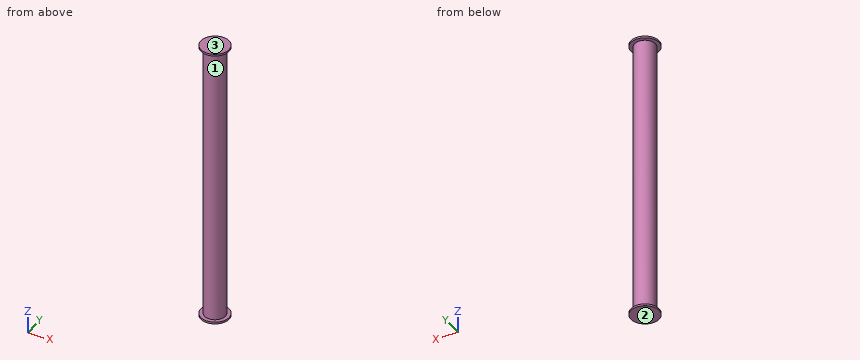
from build123d import *

# Parameters (mm, degrees)
SKETCH1_R           = 5.5
BOSS_EXTRUDE1_DEPTH = 150
SKETCH2_R           = 7.5
BOSS_EXTRUDE2_DEPTH = 1
SKETCH3_R           = 7.5
BOSS_EXTRUDE3_DEPTH = 1


with BuildPart() as part:
    # Sketch1 → Boss-Extrude1 (new body)
    with BuildSketch(Plane.XY):
        Circle(SKETCH1_R)
    extrude(amount=BOSS_EXTRUDE1_DEPTH)

    # Sketch2 → Boss-Extrude2 (add)
    with BuildSketch(Plane(origin=(0, 0, 0), x_dir=(-1, 0, 0), z_dir=(0, 0, -1))):
        Circle(SKETCH2_R)
    extrude(amount=BOSS_EXTRUDE2_DEPTH)

    # Sketch3 → Boss-Extrude3 (add)
    with BuildSketch(Plane.XY.offset(150)):
        Circle(SKETCH3_R)
    extrude(amount=BOSS_EXTRUDE3_DEPTH)


solid = part.part
Could you check a few things on this model? Use its own coordinates, in mm. Face numbers are marked on the shaded views. Give positions to 0.01 mm unless a question says otherwise; leave off trailing zeros. Order: outer loops, then holes, each group sorted by start corner. A loop starts at its lowest first (then second) coordinate and runs counter-clockwise, first axis right, second up. Notation, with made-up numbers: (38.25, -6.5) - (51.25, -6.5) arc R18 ccw to (51.25, 0.5) - close; hole circle Ø2 at (83, -8.5). An arc over 180 degrees is marked (long way). One line per item, written item: value. Start each with the question number.
1. For P1, Ø1.5, axis at y = 5.5, z = 22, coming from the -X side; P2, Ø2, axis at x = 2.5, z = 28.5, coming from the +Y side; P3, Ø4, axis at x = -5.5, z = 113, coming from the +Y side, each with a flat end and sliding along its axis, tell me the tip position at first contact or that it passes through.
2. If I drill on probe 1 along Z at (x, y) = (6.5, 1.75); probe 2 along Y at (x, z) = (0, 45); probe 3 along X at (y, z) = (3.5, 118.5), over which ranges is the centre line in solid material (lowest first)?
3. Thinking about a two-plate mould opening in Z: for the marked faces 1, 2 and 3, which applies, +Z half, -Z half, draft (parallel to the pull), parting line (faces both ways), or undercut?
4. Imagine slicing it at C-C on z = 139. List the corners of the cut face in (x, y) for me, plus the area to 3 significant figures.
5. Imagine slicing it at A-A on x = 0. List the corners of the cut face in (y, z) for me.
Values:
1. P1: x = -2.77
1. P2: y = 5.29
1. P3: y = 4.24
2. probe 1: -1 to 0, 150 to 151
2. probe 2: -5.5 to 5.5
2. probe 3: -4.24 to 4.24
3. face 1: undercut
3. face 2: -Z half
3. face 3: +Z half
4. outline: circle Ø11 at (0, 0)
4. area: 95.0 mm²
5. outline: (-7.5, -1) - (7.5, -1) - (7.5, 0) - (5.5, 0) - (5.5, 150) - (7.5, 150) - (7.5, 151) - (-7.5, 151) - (-7.5, 150) - (-5.5, 150) - (-5.5, 0) - (-7.5, 0) - close
